Autodesk Inventor part; units mm, degrees
ref_plane "Work Plane1" through (29, 0, 0) normal (0, -1, 0) x (1, 0, 0)
ref_plane "YZ Plane" through (0, 0, 0) normal (1, 0, 0) x (0, 1, 0)
ref_plane "XZ Plane" through (0, 0, 0) normal (0, 1, 0) x (-1, 0, 0)
sketch "Sketch1" plane through (0, 0, 0) normal (0, 0, 1) x (1, 0, 0)
  line L0 (-0.7366, 0) -> (9.525, 0)
  line L1 (9.525, 0) -> (9.525, 1.2573)
  line L2 (9.525, 1.2573) -> (1.323, 1.2573)
  line L3 (1.323, 1.2573) -> (0.0001, 1.2573)
  line L4 (0.0001, 1.2573) -> (0, 1.2573)
  line L5 (0, 1.2573) -> (0, 2.0447)
  line L6 (0, 2.0447) -> (-2.5146, 2.0447)
  line L7 (-2.5146, 2.0447) -> (-2.5146, 1.1438)
  line L8 (-2.5146, 1.1438) -> (-1.397, 1.1438)
  line L9 (-1.397, 1.1438) -> (-0.7366, 0)
  line L10 (-4.9225, 0) -> (11.9329, 0)
  line L11 (0, -0.4089) -> (0, 2.4536)
  line L12 (1.323, 1.2573) -> (0, 1.2573) construction
  dimension "d1" = 8.202
  dimension "d2" = 1.3229
  dimension "d3" = 2.5146
  dimension "d4" = 1.1176
  dimension "d5" = 60
  dimension "d6" = 2.5146
  dimension "d7" = 2.5146
  dimension "d8" = 2.2877
  dimension "d9" = 4.0894
  dimension "d26" = 9.525
revolve "Body" add sketch "Sketch1" angle 360 about axis through (-0.7366, 0, 0) along (1, 0, 0)
sketch "Sketch2" plane through (-2.5146, 0, 0) normal (-1, 0, 0) x (0, 0, 1)
  circle A0 centre (0, 0) radius 1.1438
  line L0 (0, -2.8626) -> (0, 2.8626)
  line L1 (-2.8626, 0) -> (2.8626, 0)
  line L2 (1.1438, 0) -> (0.5719, -0.9906)
  line L3 (0.5719, -0.9906) -> (-0.5719, -0.9906)
  line L4 (-0.5719, -0.9906) -> (-1.1438, 0)
  line L5 (-1.1438, 0) -> (-0.5719, 0.9906)
  line L6 (-0.5719, 0.9906) -> (0.5719, 0.9906)
  line L7 (0.5719, 0.9906) -> (1.1438, 0)
  point P0 (0, 0)
extrude "Slot" add sketch "Sketch2" against normal up to next contours L7 A0 | A0 L2 | L6 L0 A0 | A0 L0 L3 | L0 L6 A0 | A0 L3 L0 | L4 A0 | A0 L5
fillet "Fillet1" radius 0.2032 1 edges at (-2.5146, -2.0447, 0)
thread "Thread"
chamfer "Chamfer1" distance 0.3162 distance2 0.3162 1 edges at (9.525, -1.2573, 0) measured on face at (9.525, 0.2955, 0.1278)
ref_plane "Work Plane1" through (29, 0, 0) normal (0, -1, 0) x (1, 0, 0)
fillet "Fillet2" radius 0.1016 1 edges at (0.0001, -1.2573, 0)
equation "\"d1\" = GEL"
equation "\"d3\" = KOH"
equation "\"d4\" = INTI"
equation "\"d6\" = GD"
equation "\"d7\" = BDM"
equation "\"d8\" = 1.1547 * SW"
equation "\"d9\" = KOD"
equation "\"d26\" = NLG"
equation "\"d30\" = R"
equation "\"d17\" = RR"
equation "\"d13\" = GEL"
equation "\"d15\" = -0.5 * SPD + 0.5 * GD"
equation "\"d16\" = GUL"
equation "\"GD\" = 2.5146"
equation "\"NLG\" = 9.525"
equation "\"GEL\" = 8.20197"
equation "\"KOD\" = 4.0894"
equation "\"KOH\" = 2.5146"
equation "\"INTI\" = 1.1176"
equation "\"GAL\" = 1.32283"
equation "\"GUL\" = 0.31623"
equation "\"BDM\" = 2.5146"
equation "\"SW\" = 1.9812"
equation "\"RR\" = 0.2032"
equation "\"SPD\" = 1.88214"
equation "\"R\" = 0.1016"
equation "\"PHH\" = 0.0762"
equation "\"GD1\" = SPD"
equation "\"THREADDIA\" = 2.5146"
equation "\"FAWI\" = 45deg"
equation "\"KOH1\" = 2.2606"
equation "\"NND\" = 2.5146"
equation "\"TOA\" = 30deg"
equation "\"E0\" = 1.155 * SW"
properties part number "ANSI B18.3 - No. 3 - 48 UNC - 3/8 HS HCS"
Verification items for the finished model (mm, model axes). A direction names the side the tool comes from. Coordinates: 2 decimals unless noted, no trailing zeros. Order: outer loops, then holes, each group sorted by start corner. A loop starts at its lowest first (then second) coordinate and runs counter-clockwise, first axis right, second up. Notation, with made-up numbers: M 26,54 L 48,54 A29 cw 48,75 Z; hole C 37,-12.75 d9. An arc over 180 degrees is marked long. One line per item, written item: value. Start each with the question number.
Item 1: Sectioned sample at A-A (x = 3). Enter the section's corners in (y, z), then the cut area to 3 significant figures.
Item 2: Scan lines: probe 1 along Y at (x, z) = (-1.75, -0.7); probe 2 along Y at (x, z) = (-1.25, 0.4); probe 3 along X at (y, z) = (-0.2, -1.35). Record each from-to range of solid material in increasing order.
Item 3: Access from +Z, -Z, +X, -X, +Y, -Y to the whole of each face (thin tool, end or side, straight path). Record for faces 1 (the flat face through (-1.92, 0.502, 0.854)), 2 (the cylindrical face through (4.59, -0.27, 1.23)), 3 (the flat face through (9.525, 0, 0)).
Item 4: Mould release check, pull along Z, two halves, no side actions. Record for faces 4 (the flat face through (-2.515, -1, 1)), 5 (the conical face through (-0.778, -0.009, -0.071)), 6 (the cylindrical face through (-1.17, 1.95, -0.61)): released by +Z, released by -Z, zero draft, split by the parting line, or undercut.
Item 5: Gauge pin test, flat ends, axial feed: pin 1 (1.5 mm diameter, centred on x = 2, z = -1, fed in from -Y); pin 2 (1.5 mm diameter, centred on x = 1.5, y = 1, fed in from +Z); pin 3 (1 mm diameter, centred on x = 0, y = 1, fed in from +Z). Record the tip position at first contact, or that the pin passes through.
Conclusion:
1. outline: C 0,0 d2.51
1. area: 4.97 mm^2
2. probe 1: y = -1.92 to -0.77, 0.77 to 1.92
2. probe 2: y = -2.01 to -0.79, 0.79 to 2.01
2. probe 3: x = -2.51 to 0
3. face 1: -X
3. face 2: +X
3. face 3: +Z, -Z, +X, +Y, -Y
4. face 4: zero draft
4. face 5: undercut
4. face 6: split by the parting line
5. pin 1: stops at y = -1.23
5. pin 2: stops at z = 1.23
5. pin 3: stops at z = 1.98
